Work out the finished part from the listing and answer in its coordinate system (mm). Give positions to 0.01 mm unless a question says otherwise; leave off trailing zeros. Order: outer loops, then holes, each group sorted by start corner. A loop starts at its lowest first (then second) coordinate and runs counter-clockwise, first axis right, second up. Notation, with made-up numbers: (52.25, -22) - (69.25, -22) arc R31 ccw to (69.25, 6) - close; hole circle Ø7 at (1, -31). An arc over 180 degrees is marked (long way). Write each question's results on one line, items separated by ' | '.
from build123d import *

# Parameters (mm, degrees)
F0_W     = 600
F0_H     = 147.5
F1_DEPTH = 2
F2_R     = 2
F3_R     = 19.05
F4_DEPTH = 25


with BuildPart() as f1:
    # F0 (on Right) → F1 (new body)
    with BuildSketch(Plane.YZ):
        Rectangle(F0_W, F0_H)
    extrude(amount=F1_DEPTH)

    # F2
    f2_edges = [f1.edges().sort_by_distance(p)[0] for p in [
        (1, -300, -73.75),
        (1, 300, -73.75),
    ]]
    fillet(f2_edges, radius=F2_R)

    # F3 (on face) → F4 (cut)
    with BuildSketch(Plane.YZ.offset(2)):
        with Locations((-70, -58.75)):
            Circle(F3_R)
    extrude(amount=-F4_DEPTH, mode=Mode.SUBTRACT)


solid = f1.part
1. A cutting plane is placed at A-A, the plane z = -58.75. Write down the section's boundary in (x, y).
Answer list:
outline: (0, -300) - (2, -300) - (2, -89.05) - (0, -89.05) - close; (0, -50.95) - (2, -50.95) - (2, 300) - (0, 300) - close
2. A cutting plane is placed at B-B, the plane y = -70. Write down the section's boundary in (x, z), then the cut area to 3 significant figures.
Answer list:
outline: (0, -39.7) - (2, -39.7) - (2, 73.75) - (0, 73.75) - close | area: 227 mm^2
3. Straight lines are drawn through the part: line 1 (Y direction, x = 1.2, z = -58.75); line 2 (Z direction, x = 1.35, y = -70); line 3 (Z direction, x = 1.1, y = -82). For each, find the intervals that lie inside material, in ascending order. Write a range as [from, to].
Answer list:
line 1: [-300, -89.05], [-50.95, 300] | line 2: [-39.7, 73.75] | line 3: [-73.75, -73.55], [-43.95, 73.75]
